Check sheet for the modelled part. Datum: model origin and axes. Units: mm. A direction names the side the tool comes from. Coordinates: 2 decimals unless noted, no trailing zeros. Loops run counter-clockwise (first coordinate to the right, second up) from the corner with the lowest first, then second, coordinate; pieces in that order, holes last.
```python
from build123d import *

# Parameters (mm, degrees)
F0_R     = 1.5
F1_DEPTH = 1.8
F2_DEPTH = 10
F3_R     = 1.2
F4_DEPTH = 264.001


with BuildPart() as f1:
    # F0 (on Right) → F1 (new body)
    with BuildSketch(Plane.YZ):
        Polygon((-132, -60), (132, -60), (132, 60), (-132, 60), (-132, 45), (-130.2, 45), (-130.2, 40), (-130.2, 35), (-132, 35), (-132, -35), (-130.2, -35), (-130.2, -40), (-130.2, -45), (-132, -45), align=None)
        with Locations((20, -28)):
            Circle(F0_R, mode=Mode.SUBTRACT)
        with Locations((83, -28)):
            Circle(F0_R, mode=Mode.SUBTRACT)
        with Locations((-109, 4)):
            Circle(F0_R, mode=Mode.SUBTRACT)
        with Locations((-19, 4)):
            Circle(F0_R, mode=Mode.SUBTRACT)
        with Locations((-109, 39)):
            Circle(F0_R, mode=Mode.SUBTRACT)
        with Locations((-19, 39)):
            Circle(F0_R, mode=Mode.SUBTRACT)
        with Locations((2, 4)):
            Circle(F0_R, mode=Mode.SUBTRACT)
        with Locations((90, 4)):
            Circle(F0_R, mode=Mode.SUBTRACT)
        with Locations((2, 39)):
            Circle(F0_R, mode=Mode.SUBTRACT)
        with Locations((90, 39)):
            Circle(F0_R, mode=Mode.SUBTRACT)
        with Locations((113.8, 54)):
            Circle(F0_R, mode=Mode.SUBTRACT)
        Polygon((-130.2, 45), (-132, 45), (-132, 35), (-130.2, 35), (-130.2, 40), align=None)
        Polygon((-132, -35), (-132, -45), (-130.2, -45), (-130.2, -40), (-130.2, -35), align=None)
    extrude(amount=F1_DEPTH)

    # F0 (on Right) → F2 (join)
    with BuildSketch(Plane.YZ):
        Polygon((-130.2, 45), (-132, 45), (-132, 35), (-130.2, 35), (-130.2, 40), align=None)
        Polygon((-132, -35), (-132, -45), (-130.2, -45), (-130.2, -40), (-130.2, -35), align=None)
    extrude(amount=F2_DEPTH)

    # F3 (on face) → F4 (cut, through all)
    with BuildSketch(Plane.XZ.offset(132)):
        with Locations((6, 40)):
            Circle(F3_R)
        with Locations((6, -40)):
            Circle(F3_R)
    extrude(amount=-F4_DEPTH, mode=Mode.SUBTRACT)


solid = f1.part
```
1) Section check B-B on y = -46. Enter the section's corners in (x, z).
Answer sheet:
outline: (0, -60) - (1.8, -60) - (1.8, 60) - (0, 60) - close
2) Depth check by flat-ended pin: pin 1 (10 mm diameter, centred on y = 51.5, z = 31.5, fed in from +X); pin 2 (1.9 mm diameter, centred on x = 6, z = -40, fed in from -Y); pin 3 (1.4 mm diameter, centred on x = 4.5, y = -131.5, fed in from +Z); pin 4 (6 mm diameter, centred on x = 2.5, y = -47, fed in from +Z). Enter the tip coordinate at first touch or a pass-through.
Answer sheet:
pin 1: stops at x = 1.8
pin 2: passes through
pin 3: stops at z = 45
pin 4: stops at z = 60
3) Scan lines: line 1 (Z direction, x = 0.95, y = -19); line 2 (X direction, y = -46, z = 23.5); line 3 (Y direction, x = 5, z = -37). Record each from-to range of solid material in increasing order.
Answer sheet:
line 1: z = -60 to 2.5, 5.5 to 37.5, 40.5 to 60
line 2: x = 0 to 1.8
line 3: y = -132 to -130.2
4) Set-up check for faces 1 (the flat face through (5, -130.2, -39)), 2 (the flat face through (1.6, -132, 0.8)): record each of +Z, -Z, +X, -X, +Y, -Y from which the full face is reachable in a straight line by a thin tool's end or side.
Answer sheet:
face 1: +Z, -Z, +X, +Y
face 2: +Z, -Z, +X, -X, -Y
5) Section check A-A on z = -8. Enter the section's corners in (x, y).
Answer sheet:
outline: (0, -132) - (1.8, -132) - (1.8, 132) - (0, 132) - close
